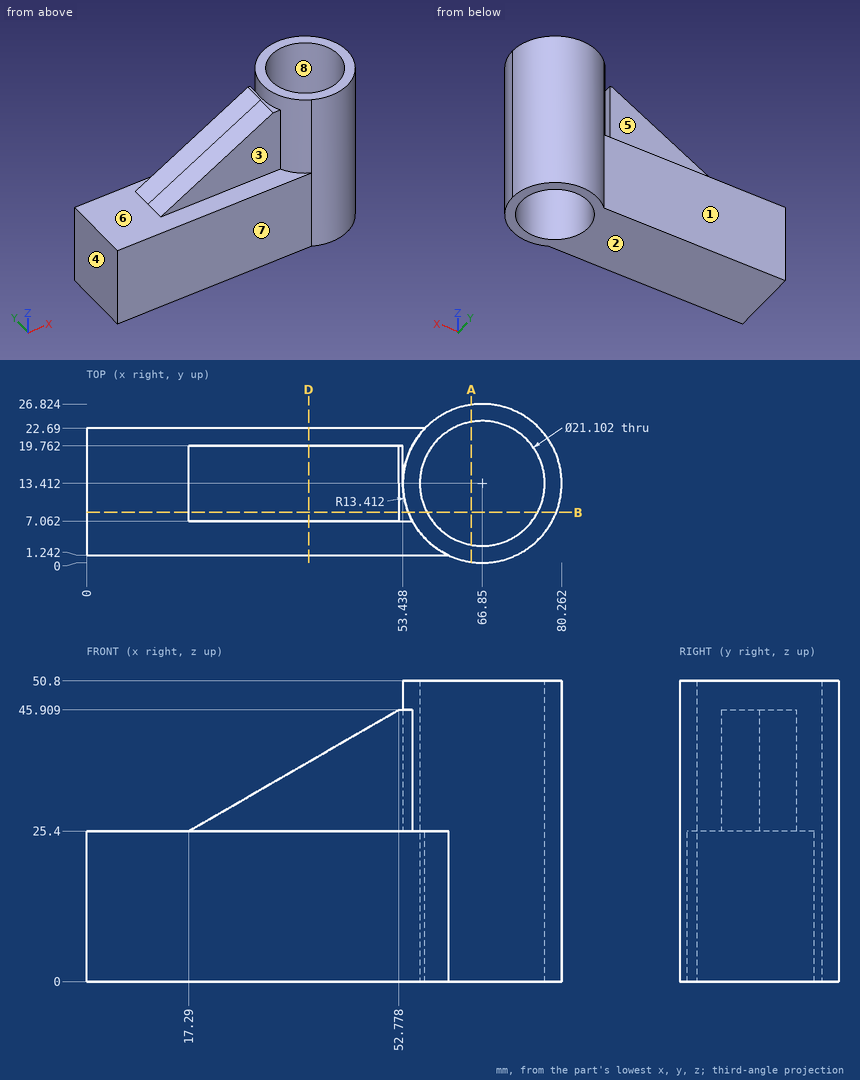
Can you work these out from the drawing? Everything is in mm from the part's minimum corner. A direction names the side the tool comes from. Round coordinates to 2 decimals unless told otherwise and drop trailing zeros. Loops run counter-clockwise (first coordinate to the right, second up) from the corner with the lowest first, then second, coordinate; pieces in that order, holes last. Notation, with made-up numbers: (-11, -19) - (26, -19) arc R16 ccw to (26, -4) - close; hole circle Ø5 at (47.5, 43.25). An arc over 180 degrees is marked (long way). Answer as CSV lines item,"result".
1. For pin 1 Ø6 at (x, z) = (27.5, 32.5) entering from -Y; pin 2 Ø3 at (y, z) = (3.5, 15.5) entering from +X (1 decimal); pin 3 Ø3 at (x, y) = (52, 15.5) entering from +Z, each with a flat end and sliding along its axis, tell me the tip position at first contact or that it passes through.
Filled in:
pin 1,"stops at y = 7.06"
pin 2,"stops at x = 77.3"
pin 3,"stops at z = 45.91"
2. I want a section at B-B on y = 8.5. List the corners of the cut face in (x, z) for me, then the cut area to 3 significant figures.
Filled in:
outline,"(0, 0) - (57.51, 0) - (57.51, 50.8) - (54.37, 50.8) - (54.37, 45.91) - (52.78, 45.91) - (17.29, 25.4) - (0, 25.4) - close; (76.19, 0) - (79.33, 0) - (79.33, 50.8) - (76.19, 50.8) - close"
area,"2,100 mm^2"
3. On a 3-axis mill with a long thin cutter (end or side, diameter ignored), from which of +Z, -Z, +X, -X, +Y, -Y can I reach the whole of each face in a straight line? I mean the marked faces 1, 2, 3, 4 and 5. Say none if no direction works.
Filled in:
face 1,"+Z, -Z, -X, +Y"
face 2,"-Z, +X, -X, +Y, -Y"
face 3,"+Z, -X, -Y"
face 4,"+Z, -Z, -X, +Y, -Y"
face 5,"+Z, -X, +Y"
4. We'd pull the mould along Y, two halves only. Please class the marked faces 6, 7 and 8: +Y half, -Y half, draft (parallel to the pull), parting line (faces both ways), or undercut.
Filled in:
face 6,"draft"
face 7,"-Y half"
face 8,"undercut"
5. I want a section at A-A on x = 65. List the corners of the cut face in (y, z) for me (1 decimal), then the cut area to 3 significant figures.
Filled in:
outline,"(0.1, 0) - (3, 0) - (3, 50.8) - (0.1, 50.8) - close; (23.8, 0) - (26.7, 0) - (26.7, 50.8) - (23.8, 50.8) - close"
area,"294 mm^2"
6. Please list where these lines run through material, in increasing order: line 1 along X through (y, z) = (17.5, 41) (1 decimal); line 2 along Y through (x, z) = (18, 16.5); line 3 along Y through (x, z) = (49, 34). Write a range as [from, to].
Filled in:
line 1,"x = [44.3, 53.4], [54.1, 57.1], [76.6, 79.6]"
line 2,"y = [1.24, 22.69]"
line 3,"y = [7.06, 19.76]"
7. I want a section at D-D on x = 37.5. List the corners of the cut face in (y, z) for me.
Filled in:
outline,"(1.24, 0) - (22.69, 0) - (22.69, 25.4) - (19.76, 25.4) - (19.76, 37.08) - (7.06, 37.08) - (7.06, 25.4) - (1.24, 25.4) - close"
